Build history of the part. All positions in model axes, mm. Face numbers are marked on the shaded views. A direction names the side the tool comes from. Give positions to 0.01 mm unless a question says otherwise; leave off trailing zeros. Write each loop counter-clockwise with the first axis right and the second up, starting at its lowest first coordinate (ties: lowest second). Pieces come first, ordered by that corner, then holes.
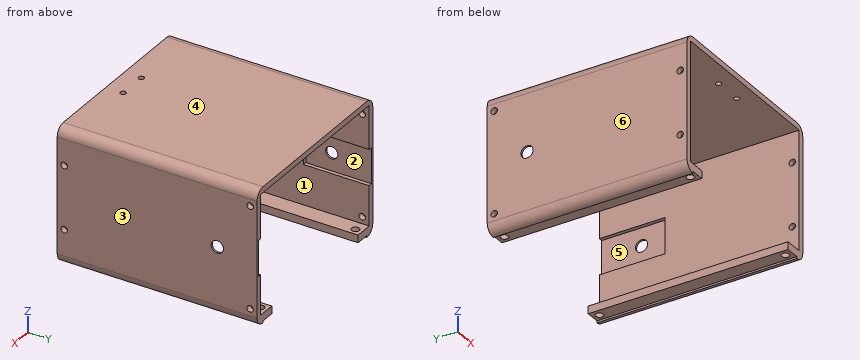
from build123d import *

# Parameters (mm, degrees)
BOSS_EXTRUDE1_DEPTH     = 104.887
SKETCH2_R               = 1.7
CUT_EXTRUDE1_DEPTH      = 148.161043653
SKETCH6_R               = 1.7
CUT_EXTRUDE9_DEPTH      = 148.161043653
SKETCH3_9_R             = 3.2
CUT_EXTRUDE4_DEPTH      = 148.161043653
SKETCH4_R               = 2
CUT_EXTRUDE5_DEPTH      = 4
SKETCH5_R               = 1.43
CUT_EXTRUDE6_DEPTH      = 136.417475863
MIRROR9_COPY_1_SKETCH_R = 2
MIRROR9_COPY_1_DEPTH    = 4
CUT_EXTRUDE7_START      = -1
SKETCH3_10_W            = 10.4
SKETCH3_10_H            = 14.6
SKETCH3_10_H_2          = 12.6
SKETCH3_10_R            = 3.2
SKETCH3_10_R_2          = 1
CUT_EXTRUDE7_DEPTH      = 2
CUT_EXTRUDE8_START      = -94
SKETCH3_W               = 10.4
SKETCH3_H               = 14.6
SKETCH3_H_2             = 12.6
SKETCH3_R               = 3.2
SKETCH3_R_2             = 1
CUT_EXTRUDE8_DEPTH      = 2


with BuildPart() as part:
    # Sketch1 → Boss-Extrude1 (new body)
    with BuildSketch(Plane(origin=(0, 0, 0), x_dir=(1, 0, 0), z_dir=(0, 1, 0))):
        with BuildLine():
            ThreePointArc((-48.5, -30.3), (-47.035533906, -33.835533906), (-43.5, -35.3))
            Line((-43.5, -35.3), (43.5, -35.3))
            ThreePointArc((43.5, -35.3), (47.035533906, -33.835533906), (48.5, -30.3))
            Line((48.5, -30.3), (48.5, 30.3))
            ThreePointArc((48.5, 30.3), (47.035533906, 33.835533906), (43.5, 35.3))
            Line((43.5, 35.3), (43.5, 34.3))
            Line((43.5, 34.3), (36.2, 34.3))
            Line((36.2, 34.3), (36.2, 30.3))
            Line((36.2, 30.3), (45.5, 30.3))
            Line((45.5, 30.3), (45.5, -32.3))
            Line((45.5, -32.3), (-45.5, -32.3))
            Line((-45.5, -32.3), (-45.5, 30.3))
            Line((-45.5, 30.3), (-36.2, 30.3))
            Line((-36.2, 30.3), (-36.2, 34.3))
            Line((-36.2, 34.3), (-43.5, 34.3))
            Line((-43.5, 34.3), (-43.5, 35.3))
            ThreePointArc((-43.5, 35.3), (-47.035533906, 33.835533906), (-48.5, 30.3))
            Line((-48.5, 30.3), (-48.5, -30.3))
        make_face()
    extrude(amount=BOSS_EXTRUDE1_DEPTH)

    # Sketch2 → Cut-Extrude1 (cut, through all)
    with BuildSketch(Plane(origin=(48.5, 0, 0), x_dir=(0, 0, -1), z_dir=(1, 0, 0))):
        with Locations((16.65, 3.65)):
            Circle(SKETCH2_R)
        with Locations((-16.65, 3.65)):
            Circle(SKETCH2_R)
    extrude(amount=-CUT_EXTRUDE1_DEPTH, mode=Mode.SUBTRACT)

    # Sketch6 → Cut-Extrude9 (cut, through all)
    with BuildSketch(Plane(origin=(48.5, 0, 0), x_dir=(0, 0, -1), z_dir=(1, 0, 0))):
        with Locations((-26.65, 101.237)):
            Circle(SKETCH6_R)
    cut_extrude9 = extrude(amount=-CUT_EXTRUDE9_DEPTH, mode=Mode.SUBTRACT)

    # Mirror11: Cut-Extrude9 across plane
    add(cut_extrude9.mirror(Plane.XY), mode=Mode.SUBTRACT)

    # Sketch3<9> → Cut-Extrude4 (cut, through all)
    with BuildSketch(Plane.ZY.offset(48.5)):
        with Locations((0, 83.987)):
            Circle(SKETCH3_9_R)
    extrude(amount=-CUT_EXTRUDE4_DEPTH, mode=Mode.SUBTRACT)

    # Sketch4 → Cut-Extrude5 (cut)
    with BuildSketch(Plane(origin=(0, 0, -34.3), x_dir=(-1, 0, 0), z_dir=(0, 0, -1))):
        with Locations((39.85, 3.65)):
            Circle(SKETCH4_R)
    cut_extrude5 = extrude(amount=-CUT_EXTRUDE5_DEPTH, mode=Mode.SUBTRACT)

    # Mirror7: Cut-Extrude5 across plane
    add(cut_extrude5.mirror(Plane(origin=(0, 0, 0), x_dir=(0, 0, 1), z_dir=(1, 0, 0))), mode=Mode.SUBTRACT)

    # Sketch5 → Cut-Extrude6 (cut, through all)
    with BuildSketch(Plane.XY.offset(35.3)):
        with Locations((-7.625, 9.05)):
            Circle(SKETCH5_R)
        with Locations(Location((7.625, 9.05, 0), (0, 0, 180))):
            Circle(SKETCH5_R)
    extrude(amount=-CUT_EXTRUDE6_DEPTH, mode=Mode.SUBTRACT)

    # Mirror9: Cut-Extrude5 across plane
    add(cut_extrude5.mirror(Plane.ZX.offset(52.4435)), mode=Mode.SUBTRACT)

    # Mirror9 copy 1 sketch → Mirror9 copy 1 (cut)
    with BuildSketch(Plane(origin=(0, 104.887, -34.3), x_dir=(1, 0, 0), z_dir=(0, 0, -1))):
        with Locations((39.85, 3.65)):
            Circle(MIRROR9_COPY_1_SKETCH_R)
    extrude(amount=-MIRROR9_COPY_1_DEPTH, mode=Mode.SUBTRACT)

    # Sketch3<10> → Cut-Extrude7 (cut)
    # profile 1 of 8: a face of its own
    with BuildSketch(Plane.ZY.offset(48.5).offset(CUT_EXTRUDE7_START)):
        Polygon((-5.2, 77.687), (-5.2, 90.287), (-5.2, 104.887), (-9.4, 104.887), (-9.4, 77.687), align=None)
    # profile 2 of 8: a face of its own
    with BuildSketch(Plane.ZY.offset(48.5).offset(CUT_EXTRUDE7_START)):
        Polygon((5.2, 104.887), (5.2, 90.287), (5.2, 77.687), (9.4, 77.687), (9.4, 104.887), align=None)
    # profile 3 of 8: a face of its own
    with BuildSketch(Plane.ZY.offset(48.5).offset(CUT_EXTRUDE7_START)):
        with Locations((0, 97.587)):
            Rectangle(SKETCH3_10_W, SKETCH3_10_H)
    # profile 4 of 8: a face of its own
    with BuildSketch(Plane.ZY.offset(48.5).offset(CUT_EXTRUDE7_START)):
        Polygon((-9.4, 70.387), (9.4, 70.387), (9.4, 77.687), (5.2, 77.687), (-5.2, 77.687), (-9.4, 77.687), align=None)
    # profile 5 of 8: a face of its own
    with BuildSketch(Plane.ZY.offset(48.5).offset(CUT_EXTRUDE7_START)):
        with Locations((0, 83.987)):
            Rectangle(SKETCH3_10_W, SKETCH3_10_H_2)
        with Locations((0, 83.987)):
            Circle(SKETCH3_10_R, mode=Mode.SUBTRACT)
        with Locations((0, 79.487)):
            Circle(SKETCH3_10_R_2, mode=Mode.SUBTRACT)
        with Locations((0, 88.487)):
            Circle(SKETCH3_10_R_2, mode=Mode.SUBTRACT)
    # profile 6 of 8: a face of its own
    with BuildSketch(Plane.ZY.offset(48.5).offset(CUT_EXTRUDE7_START)):
        with Locations((0, 79.487)):
            Circle(SKETCH3_10_R_2)
    # profile 7 of 8: a face of its own
    with BuildSketch(Plane.ZY.offset(48.5).offset(CUT_EXTRUDE7_START)):
        with Locations((0, 83.987)):
            Circle(SKETCH3_10_R)
    # profile 8 of 8: a face of its own
    with BuildSketch(Plane.ZY.offset(48.5).offset(CUT_EXTRUDE7_START)):
        with Locations((0, 88.487)):
            Circle(SKETCH3_10_R_2)
    extrude(amount=-CUT_EXTRUDE7_DEPTH, mode=Mode.SUBTRACT)

    # Sketch3 → Cut-Extrude8 (cut)
    # profile 1 of 8: a face of its own
    with BuildSketch(Plane.ZY.offset(48.5).offset(CUT_EXTRUDE8_START)):
        Polygon((-5.2, 77.687), (-5.2, 90.287), (-5.2, 104.887), (-9.4, 104.887), (-9.4, 77.687), align=None)
    # profile 2 of 8: a face of its own
    with BuildSketch(Plane.ZY.offset(48.5).offset(CUT_EXTRUDE8_START)):
        Polygon((5.2, 104.887), (5.2, 90.287), (5.2, 77.687), (9.4, 77.687), (9.4, 104.887), align=None)
    # profile 3 of 8: a face of its own
    with BuildSketch(Plane.ZY.offset(48.5).offset(CUT_EXTRUDE8_START)):
        with Locations((0, 97.587)):
            Rectangle(SKETCH3_W, SKETCH3_H)
    # profile 4 of 8: a face of its own
    with BuildSketch(Plane.ZY.offset(48.5).offset(CUT_EXTRUDE8_START)):
        with Locations((0, 83.987)):
            Rectangle(SKETCH3_W, SKETCH3_H_2)
        with Locations((0, 83.987)):
            Circle(SKETCH3_R, mode=Mode.SUBTRACT)
        with Locations((0, 79.487)):
            Circle(SKETCH3_R_2, mode=Mode.SUBTRACT)
        with Locations((0, 88.487)):
            Circle(SKETCH3_R_2, mode=Mode.SUBTRACT)
    # profile 5 of 8: a face of its own
    with BuildSketch(Plane.ZY.offset(48.5).offset(CUT_EXTRUDE8_START)):
        with Locations((0, 88.487)):
            Circle(SKETCH3_R_2)
    # profile 6 of 8: a face of its own
    with BuildSketch(Plane.ZY.offset(48.5).offset(CUT_EXTRUDE8_START)):
        with Locations((0, 83.987)):
            Circle(SKETCH3_R)
    # profile 7 of 8: a face of its own
    with BuildSketch(Plane.ZY.offset(48.5).offset(CUT_EXTRUDE8_START)):
        with Locations((0, 79.487)):
            Circle(SKETCH3_R_2)
    # profile 8 of 8: a face of its own
    with BuildSketch(Plane.ZY.offset(48.5).offset(CUT_EXTRUDE8_START)):
        Polygon((-9.4, 70.387), (9.4, 70.387), (9.4, 77.687), (5.2, 77.687), (-5.2, 77.687), (-9.4, 77.687), align=None)
    extrude(amount=-CUT_EXTRUDE8_DEPTH, mode=Mode.SUBTRACT)


solid = part.part
(1) Saw through at D-D, the plane y = 50.5. List the corners of the cut face in (x, z).
(2) Saw through at A-A, the plane z = 0. List the corners of the cut face in (x, y).
(3) Probe line 1 (X direction, y = 93.5, z = -18); line 2 (Y direction, x = 39.85, z = -31.9); line 3 (Y direction, x = 47.55, z = -16.65). List the from-to ranges inside material, lowest first.
(4) Drop flat-ended pins along their axis: pin 1 (2 mm diameter, centred on y = 67.5, z = -31.5, fed in from -X); pin 2 (1.6 mm diameter, centred on x = -46.5, z = 2.5, fed in from +Y); pin 3 (1 mm diameter, centred on x = -46.5, y = 81, fed in from +Z); pin 4 (8 mm diameter, centred on x = 40.5, y = 59, fed in from -Z). Give the stop position or say it passes through.
(5) Mould opens along X. For the marked faces 3, 4, 5 and 6 say: +X half, -X half, draft (parallel to the pull), parting line (faces both ways), or undercut.
(6) Saw through at C-C, the plane z = -11. List the corners of the cut face in (x, y), plus the area to 3 significant figures.
(7) 3-axis set-ups, long thin cutter, end or side, ignore diameter. For the marked faces 1 and 2: which of +Z, -Z, +X, -X, +Y, -Y reach the whole face in a straight line?
(8) Saw through at B-B, the plane x = -39.85. List the corners of the cut face in (y, z).
Computed values:
1. outline: (-48.5, -30.3) arc R5 ccw to (-43.5, -35.3) - (-43.5, -34.3) - (-36.2, -34.3) - (-36.2, -30.3) - (-45.5, -30.3) - (-45.5, 32.3) - (45.5, 32.3) - (45.5, -30.3) - (36.2, -30.3) - (36.2, -34.3) - (43.5, -34.3) - (43.5, -35.3) arc R5 ccw to (48.5, -30.3) - (48.5, 30.3) arc R5 ccw to (43.5, 35.3) - (-43.5, 35.3) arc R5 ccw to (-48.5, 30.3) - close
2. outline: (-48.5, 0) - (-45.5, 0) - (-45.5, 70.39) - (-47.5, 70.39) - (-47.5, 80.79) - (-48.5, 80.79) - close; (-48.5, 87.19) - (-47.5, 87.19) - (-47.5, 104.89) - (-48.5, 104.89) - close; (45.5, 0) - (48.5, 0) - (48.5, 80.79) - (47.5, 80.79) - (47.5, 70.39) - (45.5, 70.39) - close; (47.5, 87.19) - (48.5, 87.19) - (48.5, 104.89) - (47.5, 104.89) - close
3. line 1: x = -48.5 to -45.5, 45.5 to 48.5
3. line 2: y = 0 to 1.65, 5.65 to 99.24, 103.24 to 104.89
3. line 3: y = 0 to 1.95, 5.35 to 104.89
4. pin 1: stops at x = -48.5
4. pin 2: stops at y = 70.39
4. pin 3: stops at z = 34.63
4. pin 4: stops at z = -35.3
5. face 3: +X half
5. face 4: draft
5. face 5: undercut
5. face 6: -X half
6. outline: (-48.5, 0) - (-45.5, 0) - (-45.5, 104.89) - (-48.5, 104.89) - close; (45.5, 0) - (48.5, 0) - (48.5, 104.89) - (45.5, 104.89) - close
6. area: 629 mm2
7. face 1: +Y, -Y
7. face 2: +Y
8. outline: (0, -34.3) - (1.65, -34.3) - (1.65, -30.3) - (0, -30.3) - close; (0, 32.3) - (104.89, 32.3) - (104.89, 35.3) - (0, 35.3) - close; (5.65, -34.3) - (99.24, -34.3) - (99.24, -30.3) - (5.65, -30.3) - close; (103.24, -34.3) - (104.89, -34.3) - (104.89, -30.3) - (103.24, -30.3) - close
